Build history of the part. All positions in model axes, mm. Face numbers are marked on the shaded views. A direction names the side the tool comes from. Give positions to 0.01 mm unless a question says otherwise; leave off trailing zeros. Write each loop counter-clockwise with the first axis right and the second up, starting at its lowest first coordinate (ties: lowest second). Pieces come first, ordered by that corner, then holes. Notation, with made-up numbers: M -27,-13.5 L 17,-13.5 A12 ccw 17,6.5 Z; hole C -30,84.5 d8. An arc over 180 degrees is marked long. Return JSON: item names as keys, results as strings. Group by question number.
Q1. Flat gauge pins, fed straight in: pin 1 Ø4 at (x, y) = (3.5, 3.5) entering from -Z; pin 2 Ø1 at (y, z) = (5.5, -5) entering from -X. Where does each tip first touch, or does it go through?
Q2. Wall check: probe 1 along X at (y, z) = (7, 0); probe 2 along Z at (x, y) = (6, 1); probe 3 along Z at (x, y) = (22, 2.5). Give the ranges that are in metal, low to high.
Q3. Band-saw the part on C-C, the plane x = 9.5. Give the cut face in (y, z).
Q4. Band-saw the part on A-A, the plane x = 1. Give the cut face in (y, z), then the cut area to 3 significant figures.
Q5. Tool access for the marked faces 1 and 2: list every direction of +Z, -Z, +X, -X, +Y, -Y with a clear straight run to the whole face (end or side of a thin tool).
Q6. Band-saw the part on B-B, the plane y = 5. Count the separate pieces of the cut face and the enclosed holes in it, then the cut area to 3 significant figures.
from build123d import *

# Parameters (mm, degrees)
SKETCH2_R           = 5
SKETCH2_R_2         = 1.75
BOSS_EXTRUDE1_DEPTH = 8.5
BOSS_EXTRUDE2_DEPTH = 8.5


with BuildPart() as part:
    # Sketch2 → Boss-Extrude1 (new body)
    with BuildSketch(Plane(origin=(0, 0, 0), x_dir=(1, 0, 0), z_dir=(0, 1, 0))):
        with BuildLine():
            ThreePointArc((22, -5), (17, 0), (22, 5))
            Line((22, 5), (2e-09, 5))
            ThreePointArc((2e-09, 5), (3.535533907, 3.535533905), (5, 0))
            ThreePointArc((5, 0), (3.535533908, -3.535533904), (7e-09, -5))
            Line((7e-09, -5), (22, -5))
        make_face()
        Circle(SKETCH2_R)
        Circle(SKETCH2_R_2, mode=Mode.SUBTRACT)
        with Locations((22, 0)):
            Circle(SKETCH2_R)
        with Locations((22, 0)):
            Circle(SKETCH2_R_2, mode=Mode.SUBTRACT)
    extrude(amount=BOSS_EXTRUDE1_DEPTH)

    # Sketch3 → Boss-Extrude2 (add)
    with BuildSketch(Plane(origin=(0, 8.5, 0), x_dir=(1, 0, 0), z_dir=(0, 1, 0))):
        with BuildLine():
            Line((22, -5), (24.99, -5))
            Line((24.99, -5), (31.08, -2.029708536))
            add(Edge.make_bspline(
                [(31.08, -2.029708536), (40.738723452, 6.188270814), (53.27, 6)],
                knots=[0, 0, 0, 1, 1, 1], degree=2))
            Line((53.27, 6), (60.557013712, 9.301428655))
            Line((60.557013712, 9.301428655), (58.75, 12.87))
            add(Edge.make_bspline(
                [(11, 5), (23.320985194, 5), (28.960367737, 8.21999158), (46.060199439, 12.976683932), (52.533262276, 15.918311154), (58.75, 12.87)],
                knots=[0, 0, 0, 0, 0.362024874, 0.462024874, 1, 1, 1, 1], degree=3))
            Line((11, 5), (22, 5))
            ThreePointArc((22, 5), (27, 0), (22, -5))
        make_face()
    extrude(amount=-BOSS_EXTRUDE2_DEPTH)


solid = part.part
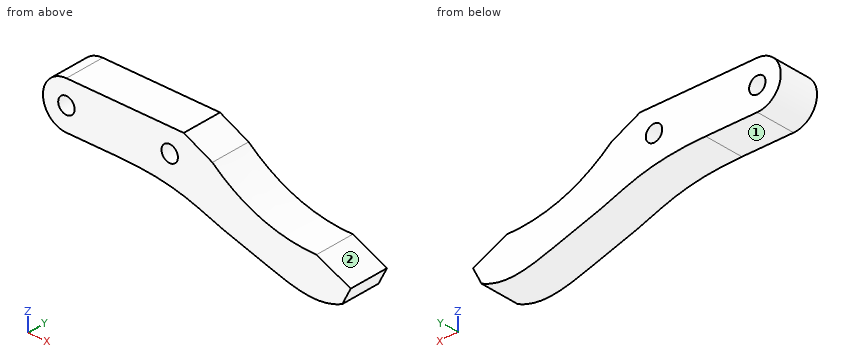
From the geometry:
{
 "1": {"pin 1": "stops at z = -5", "pin 2": "stops at x = -2.18"},
 "2": {"probe 1": "x = -5 to -1.75, 1.75 to 20.25, 23.75 to 33.69", "probe 2": "z = -5 to 5", "probe 3": "z = -5.9 to -1.75, 1.75 to 5"},
 "3": {"outline": "M 0,-5 L 8.5,-5 L 8.5,5 L 0,5 Z"},
 "4": {"outline": "M 0,-5 L 8.5,-5 L 8.5,-1.44 L 0,-1.44 Z; M 0,1.44 L 8.5,1.44 L 8.5,5 L 0,5 Z", "area": "60.6 mm^2"},
 "5": {"face 1": "-Z, -X, +Y, -Y", "face 2": "+Z, +X, +Y, -Y"},
 "6": {"separate pieces": "1", "enclosed holes": "2", "area": "569 mm^2"}
}
